The listing builds one solid part. Answer for the finished solid, in the listing's coordinates (mm). A direction names the side the tool comes from. Round coordinates to 2 decimals unless told otherwise and drop trailing zeros. Loops run counter-clockwise (first coordinate to the right, second up) from the corner with the lowest first, then second, coordinate; pieces in that order, holes last. Notation, with made-up numbers: (77, 8) -> (118, 8) arc R21 ccw to (118, 27) -> close; hole circle Ø7 at (88, -39). An arc over 180 degrees is marked (long way). Write each question's results on one line, items separated by ' | '. Start each with the question number.
(1) The part is cut by section B-B (y = 4.75). Determine the outline of the cut face in (x, z).
(2) The part is cut by section D-D (z = -15.5). Determine the outline of the cut face in (x, y), plus the area to 3 significant figures.
(3) The part is cut by section A-A (x = -5.25). Determine the outline of the cut face in (y, z).
(4) For faces 1 (the face through (3, -3, 20)), 2 (the face through (-3.755, -11.923, 10.14)), 3 (the face through (1.341, -3.233, -18.986)), determine the directions among +Z, -Z, +X, -X, +Y, -Y from which every point of the face is accessible in a straight line to the end or side of a thin tool.
(5) Straight lines are drawn through the part: probe 1 along X at (y, z) = (-0.25, 1); probe 2 along Z at (x, y) = (3.75, -5.25); probe 3 along X at (y, z) = (8.5, 16.7). For each, find the intervals that lie inside material, in ascending order.
(6) Flat-ended cylindrical pins translate along their axes: pin 1 (3 mm diameter, centred on x = 0, y = 8.5, fed in from +Z) (3 decimals); pin 2 (6 mm diameter, centred on x = 6, z = -12, fed in from +Y); pin 3 (1.5 mm diameter, centred on x = 7, y = 8.5, fed in from -Z); pin 4 (12 mm diameter, centred on x = 3.5, y = 5.5, fed in from -Z). Find the tip coordinate at first contact, or state that the pin passes through.
(7) The part is cut by section C-C (z = 2.5). Determine the outline of the cut face in (x, y).
(8) Determine the mould class of faces 4 (the face through (1.341, -3.233, 21.268)), 5 (the face through (1, -1, 32)), 6 (the face through (-0.672, 9.554, 16.696)) for opening direction X: released by +X, released by -X, zero draft, split by the parting line, or undercut.
```python
from build123d import *

# Parameters (mm, degrees)
M3X0_5_TAPPED_HOLE1_D           = 2.5
M3X0_5_TAPPED_HOLE1_DEPTH       = 6.248924226
M3X0_5_TAPPED_HOLE1_CSINK_D     = 3.05
M3X0_5_TAPPED_HOLE1_CSINK_ANGLE = 90
M3X0_5_TAPPED_HOLE1_TIP         = 0.751075774
FILLET1_R                       = 1


with BuildPart() as part:
    # Sketch1 → Revolve1 (revolve)
    with BuildSketch(Plane(origin=(0, 0, 0), x_dir=(0, 0, -1), z_dir=(1, 0, 0)), mode=Mode.PRIVATE) as revolve1_sk:
        Polygon((20, 0), (20, 3.5), (18, 3.5), (18, 12.2), (0, 12.2), (0, 12.5), (-20, 12.5), (-20, 3.5), (-22.5, 3.5), (-22.5, 2), (-32, 2), (-32, 1.2), (-24, 1.2), (-24, 0), align=None)
    revolve(revolve1_sk.sketch.rotate(Axis((0, 0, 0), (0, 0, -1)), 180), axis=Axis((0, 0, 0), (0, 0, -1)))

    # M3x0.5 Tapped Hole1
    with Locations(Plane.XY.offset(20)):
        with Locations((0, 8.5), (0, -8.5)):
            CounterSinkHole(M3X0_5_TAPPED_HOLE1_D / 2, M3X0_5_TAPPED_HOLE1_CSINK_D / 2, depth=M3X0_5_TAPPED_HOLE1_DEPTH, counter_sink_angle=M3X0_5_TAPPED_HOLE1_CSINK_ANGLE)
            with Locations((0, 0, -(M3X0_5_TAPPED_HOLE1_DEPTH + M3X0_5_TAPPED_HOLE1_TIP / 2))):  # 118° drill point
                Cone(0, M3X0_5_TAPPED_HOLE1_D / 2, M3X0_5_TAPPED_HOLE1_TIP, mode=Mode.SUBTRACT)

    # Fillet1
    fillet1_edges = [part.edges().sort_by_distance(p)[0] for p in [
        (0, 1.2, 24),
    ]]
    fillet(fillet1_edges, radius=FILLET1_R)


solid = part.part
```
Checked values:
1) outline: (-11.56, 0) -> (-11.24, 0) -> (-11.24, -18) -> (11.24, -18) -> (11.24, 0) -> (11.56, 0) -> (11.56, 20) -> (-11.56, 20) -> close
2) outline: circle Ø24.4 at (0, 0) | area: 468 mm2
3) outline: (-11.34, 0) -> (-11.01, 0) -> (-11.01, -18) -> (11.01, -18) -> (11.01, 0) -> (11.34, 0) -> (11.34, 20) -> (-11.34, 20) -> close
4) face 1: +Z | face 2: +Z, -Z | face 3: -Z
5) probe 1: x = -12.5 to 12.5 | probe 2: z = -18 to 20 | probe 3: x = -9.17 to -1.25, 1.25 to 9.17
6) pin 1: stops at z = 19.975 | pin 2: stops at y = 11.83 | pin 3: stops at z = -18 | pin 4: stops at z = -20
7) outline: circle Ø25 at (0, 0)
8) face 4: split by the parting line | face 5: zero draft | face 6: undercut
